Autodesk Inventor part; units mm, degrees
ref_plane "Work Plane4" through (0, 0, 15.6972) normal (0, 0, -1) x (-1, 0, 0)
ref_plane "YZ Plane" through (0, 0, 0) normal (1, 0, 0) x (0, 1, 0)
ref_plane "XZ Plane" through (0, 0, 0) normal (0, 1, 0) x (-1, 0, 0)
sketch "Sketch1" plane through (0, 0, 0) normal (0, 0, 1) x (1, 0, 0)
  circle A0 centre (0, 0) radius 10.541
  dimension "d0" = 21.082
extrude "Extrusion1" add sketch "Sketch1" along normal blind 2.032
ref_plane "Work Plane4" through (0, 0, 15.6972) normal (0, 0, -1) x (-1, 0, 0)
sketch "Sketch2" plane through (0, 0, 2.032) normal (0, 0, 1) x (1, 0, 0)
  circle A0 centre (0, 0) radius 9.017
  dimension "d3" = 18.034
extrude "Extrusion2" add sketch "Sketch2" along normal blind 24.003
sketch "Sketch5" plane through (0, 0, 15.6972) normal (0, 0, -1) x (-1, 0, 0)
  line L0 (0, 0) -> (9.017, 0)
  line L1 (9.017, 0) -> (9.017, 9.017)
  line L2 (9.017, 9.017) -> (0, 9.017)
  line L3 (0, 9.017) -> (0, 0)
  dimension "d16" = 9.017
  dimension "d17" = 9.017
extrude "Extrusion3" cut sketch "Sketch5" along normal blind 3.175
hole "Hole1" at (0, 0, 26.035) direction (0, 0, -1) diameter 13.97 end through all
sketch "Sketch6" plane through (0, 0, 0) normal (0, 0, -1) x (-1, 0, 0)
  line L0 (0, 0) -> (7.629, -6.3585) construction
  line L1 (0, 0) -> (9.9314, 0) construction
  circle A0 centre (7.629, -6.3585) radius 0.508
  line L2 (7.3038, -6.7487) -> (7.7626, -7.1312)
  circle A1 centre (0, 0) radius 10.541
  line L3 (7.9543, -5.9683) -> (8.4131, -6.3507)
  line L4 (0, 0) -> (7.0226, 7.0226)
  line L5 (0, 0) -> (9.9314, 0) construction
  circle A2 centre (7.0226, 7.0226) radius 0.508
  line L6 (6.6671, 7.3855) -> (7.0903, 7.8)
  line L7 (7.378, 6.6597) -> (7.8083, 7.0811)
  line L8 (10.541, 0) -> (10.541, 7.62)
  dimension "d20" = 9.9314
  dimension "d21" = 39.81
  dimension "d22" = 1.016
  dimension "d25" = 9.9314
  dimension "d26" = 45
  dimension "d27" = 1.016
  dimension "d30" = 7.62
extrude "Extrusion5" cut sketch "Sketch6" against normal through all contours A1 L7 A2 L6 | A2
sketch "Sketch7" plane through (0, 0, 26.035) normal (0, 0, 1) x (1, 0, 0)
  point P0 (0, 0)
properties part number "Piston Shaft"
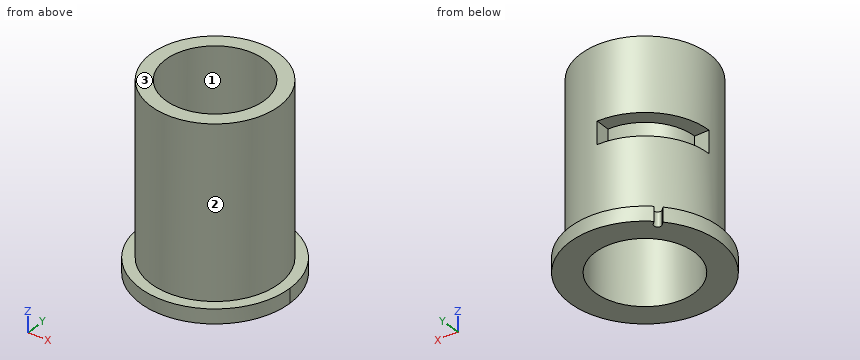
Build history of the part. All positions in model axes, mm. Face numbers are marked on the shaded views. Round coordinates to 2 decimals unless told otherwise and drop trailing zeros. Loops run counter-clockwise (first coordinate to the right, second up) from the corner with the lowest first, then second, coordinate; pieces in that order, holes last. Notation, with made-up numbers: (43.5, 6) -> (91.5, 6) arc R30 cw to (91.5, 40) -> close; hole circle Ø5 at (33.25, -19.75). An arc over 180 degrees is marked (long way). Answer in a Markdown table with one row per item.
Item 1: Drill centre lines: L1, parallel to X at y = 0, z = 16 (3 decimals); L2, parallel to Y at x = 4.25, z = 10.5. Where is each one in solid material? Low to high. Write a range as [from, to].
Answers below:
| item | result |
|---|---|
| L1 | x = [-9.017, -6.985], [6.985, 9.017] |
| L2 | y = [-7.95, -5.54], [5.54, 7.95] |
Item 2: Saw through at D-D (x = -8.5). Write the cut outline in (y, z) (3 decimals).
Answers below:
| item | result |
|---|---|
| outline | (-6.234, 0) -> (6.234, 0) -> (6.234, 2.032) -> (3.009, 2.032) -> (3.009, 12.522) -> (0, 12.522) -> (0, 15.697) -> (3.009, 15.697) -> (3.009, 26.035) -> (-3.009, 26.035) -> (-3.009, 2.032) -> (-6.234, 2.032) -> close |
Item 3: Saw through at A-A (x = 4). Write the cut outline in (y, z) (3 decimals).
Answers below:
| item | result |
|---|---|
| outline | (-9.753, 0) -> (-5.726, 0) -> (-5.726, 26.035) -> (-8.081, 26.035) -> (-8.081, 2.032) -> (-9.753, 2.032) -> close; (5.726, 0) -> (9.753, 0) -> (9.753, 2.032) -> (8.081, 2.032) -> (8.081, 26.035) -> (5.726, 26.035) -> close |
Item 4: Saw through at C-C (z = 16.25). Write the cut outline in (x, y) (3 decimals).
Answers below:
| item | result |
|---|---|
| outline | circle Ø18.034 at (0, 0); hole circle Ø13.97 at (0, 0) |
Item 5: Mould opens along Y. For the marked faces 1, 2 and 3 say: +Y half, -Y half, draft (parallel to the pull), parting line (faces both ways), or undercut.
Answers below:
| item | result |
|---|---|
| face 1 | undercut |
| face 2 | parting line |
| face 3 | draft |
Item 6: Saw through at B-B (y = 3). Write the cut outline in (x, z) (3 decimals), and give its area (3 significant figures).
Answers below:
| item | result |
|---|---|
| outline | (-10.105, 0) -> (-6.308, 0) -> (-6.308, 12.522) -> (-8.503, 12.522) -> (-8.503, 2.032) -> (-10.105, 2.032) -> close; (-8.503, 15.697) -> (-6.308, 15.697) -> (-6.308, 26.035) -> (-8.503, 26.035) -> close; (6.308, 0) -> (10.105, 0) -> (10.105, 2.032) -> (8.503, 2.032) -> (8.503, 26.035) -> (6.308, 26.035) -> close |
| area | 114 mm² |
Item 7: Pin check, flat tips, straight feed: pin 1 (8 mm diameter, centred on x = -1, y = -1, fed in from +Z); pin 2 (4 mm diameter, centred on x = 6, z = 5.5, fed in from -Y); pin 3 (1 mm diameter, centred on y = 8.5, z = 14, fed in from -X); pin 4 (5 mm diameter, centred on x = -5, z = 17.5, fed in from +Y). Stop position of each tip, or through.
Answers below:
| item | result |
|---|---|
| pin 1 | passes through |
| pin 2 | stops at y = -8.08 |
| pin 3 | stops at x = 0 |
| pin 4 | stops at y = 8.66 |
